Could you check a few things on this model? Use its own coordinates, in mm. Face numbers are marked on the shaded views. Round coordinates to 2 decimals unless told otherwise and drop trailing zeros. Loops run counter-clockwise (first coordinate to the right, second up) from the corner with the lowest first, then second, coordinate; pieces in that order, holes last. Notation, with made-up numbers: (18, 58) -> (56, 58) arc R15 ccw to (56, 79) -> close; hole circle Ø5 at (-5, 87.5). An arc over 180 degrees is marked (long way). Use CSV: the item, a comma, the result in double quotes. Start each with the question number.
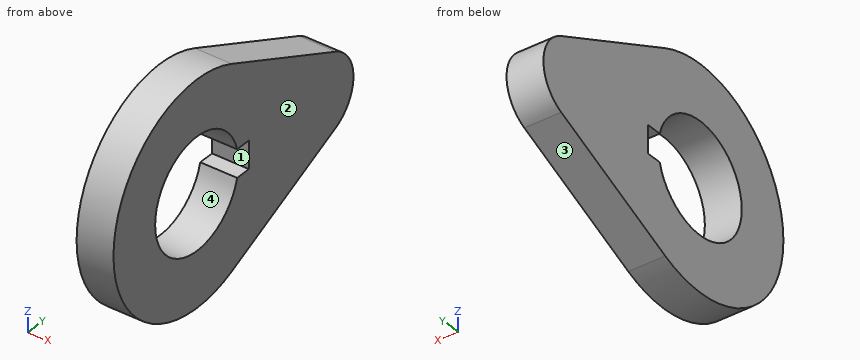
```python
from build123d import *

# Parameters (mm, degrees)
SKETCH1_R           = 38.1
SKETCH1_R_2         = 19.05
BOSS_EXTRUDE1_DEPTH = 12.7
SKETCH2_W           = 9.525
SKETCH2_H           = 9.525
CUT_EXTRUDE1_DEPTH  = 13.7
BOSS_EXTRUDE2_DEPTH = 12.7


with BuildPart() as part:
    # Sketch1 → Boss-Extrude1 (new body)
    with BuildSketch(Plane(origin=(0, 0, 0), x_dir=(0, 0, -1), z_dir=(1, 0, 0))):
        Circle(SKETCH1_R)
        Circle(SKETCH1_R_2, mode=Mode.SUBTRACT)
    extrude(amount=BOSS_EXTRUDE1_DEPTH)

    # Sketch2 → Cut-Extrude1 (cut, through all)
    with BuildSketch(Plane(origin=(12.7, 0, 0), x_dir=(0, 0, -1), z_dir=(1, 0, 0))):
        with Locations((0, 19.05)):
            Rectangle(SKETCH2_W, SKETCH2_H)
    extrude(amount=-CUT_EXTRUDE1_DEPTH, mode=Mode.SUBTRACT)

    # Sketch3 → Boss-Extrude2 (add)
    with BuildSketch(Plane(origin=(12.7, 0, 0), x_dir=(0, 0, -1), z_dir=(1, 0, 0))):
        with BuildLine():
            Line((-34.605831603, 15.938833679), (-12.7, 63.5))
            ThreePointArc((-12.7, 63.5), (0, 71.632930181), (12.7, 63.5))
            Line((12.7, 63.5), (34.605831603, 15.938833679))
            ThreePointArc((34.605831603, 15.938833679), (0, 38.1), (-34.605831603, 15.938833679))
        make_face()
    extrude(amount=-BOSS_EXTRUDE2_DEPTH)


solid = part.part
```
1. Suppose I cut it at D-D (y = 25.5). List the corners of the cut face in (x, z) for me, then the cut area to 3 significant figures.
2. We'd pull the mould along Y, two halves only. Please class the marked faces 1, 2, 3 and 4: pulls with the +Y half, pulls with the -Y half, needs draft (parallel to the pull), parting line crosses it, or undercut.
3. Suppose I cut it at A-A (x = 5.75). List the corners of the cut face in (y, z) for me.
4. If I drill on L1, parallel to Y at x = 4, z = 0; L2, parallel to Z at x = 10, y = 0; L3, parallel to Y at x = 7.5, z = 14.5, over which ranges is the centre line in solid material (lowest first)?
5. Suppose I cut it at C-C (z = 0). List the corners of the cut face in (x, y) for me.
6. Suppose I cut it at B-B (y = 0). List the corners of the cut face in (x, z) for me, then the cut area to 3 significant figures.
7. Will these pins go through, and if not, where does the flat tip stop? pin 1 (1.5 mm diameter, centred on x = 10.5, z = -7.5, fed in from +Y); pin 2 (6 mm diameter, centred on x = 6, y = 22, fed in from +Z); pin 3 (6 mm diameter, centred on x = 5.5, y = -17, fed in from -Z).
Geometry check:
1,outline,"(0, -30.2) -> (12.7, -30.2) -> (12.7, 30.2) -> (0, 30.2) -> close"
1,area,"767 mm²"
2,face 1,"undercut"
2,face 2,"needs draft"
2,face 3,"pulls with the +Y half"
2,face 4,"undercut"
3,outline,"(15.94, -34.61) -> (63.5, -12.7) arc R13.98 ccw to (63.5, 12.7) -> (15.94, 34.61) arc R38.1 ccw (long way) to start; hole (18.45, -4.76) -> (23.81, -4.76) -> (23.81, 4.76) -> (18.45, 4.76) arc R19.05 ccw (long way) to start"
4,L1,"y = -38.1 to -19.05, 23.81 to 71.63"
4,L2,"z = -38.1 to -19.05, 19.05 to 38.1"
4,L3,"y = -35.23 to -12.36, 12.36 to 59.59"
5,outline,"(0, -38.1) -> (12.7, -38.1) -> (12.7, -19.05) -> (0, -19.05) -> close; (0, 23.81) -> (12.7, 23.81) -> (12.7, 71.63) -> (0, 71.63) -> close"
6,outline,"(0, -38.1) -> (12.7, -38.1) -> (12.7, -19.05) -> (0, -19.05) -> close; (0, 19.05) -> (12.7, 19.05) -> (12.7, 38.1) -> (0, 38.1) -> close"
6,area,"484 mm²"
7,pin 1,"stops at y = 69.9"
7,pin 2,"stops at z = 33.2"
7,pin 3,"stops at z = -35.43"
